Autodesk Inventor part; units mm, degrees
ref_plane "YZ Plane" through (0, 0, 0) normal (1, 0, 0) x (0, 1, 0)
ref_plane "XZ Plane" through (0, 0, 0) normal (0, 1, 0) x (-1, 0, 0)
ref_plane "XY Plane" through (0, 0, 0) normal (0, 0, 1) x (1, 0, 0)
sketch "スケッチ2" plane through (0, 0, 0) normal (0, 1, 0) x (-1, 0, 0)
  circle A0 centre (0, 0) radius 1.5
  circle A1 centre (0, 0) radius 2.25
  circle A2 centre (0, 0) radius 2.75
  line L0 (2.75, 2.75) -> (-2.75, -2.75) construction
  line L1 (1.0066, 4.2082) -> (1.0066, -4.7182) construction
  line L2 (3.3819, 0) -> (-4.1959, 0) construction
  line L3 (-2.75, -1.5877) -> (0, -3.1754)
  line L4 (-2.1903, -1.9109) -> (0.8771, -1.9109) construction
  line L5 (-2.75, 0) -> (-2.75, -1.5877)
  line L6 (0, 3.6036) -> (0, -4.7182) construction
  line L7 (-2.75, 1.5877) -> (0, 3.1754)
  line L8 (-2.75, 0) -> (-2.75, 1.5877)
  line L9 (2.75, -1.5877) -> (0, -3.1754)
  line L10 (2.75, 0) -> (2.75, -1.5877)
  line L11 (2.75, 1.5877) -> (0, 3.1754)
  line L12 (2.75, 0) -> (2.75, 1.5877)
  dimension "d8" = 5.5
  dimension "d6" = 3
  dimension "d7" = 4.5
  dimension "d12" = 30
extrude "押し出し1" add sketch "スケッチ2" against normal blind 0.7 contours A1
extrude "押し出し2" add sketch "スケッチ2" along normal blind 2.1 contours A1 | A2 | L10 L9 A2 | A2 L11 L12 | A2 L7 L11 | L9 L3 A2 | A2 L8 L7 | L3 L5 A2
chamfer "面取り1" distance 0.2 angle 45 6 edges at (2.75, 1.05, -1.5877) (0, 1.05, -3.1754) (-2.75, 1.05, -1.5877) (-2.75, 1.05, 1.5877) (0, 1.05, 3.1754) (2.75, 1.05, 1.5877)
chamfer "面取り2" distance 0.2 angle 45 6 edges at (2.6634, 2.1, -1.5377) (0, 2.1, -3.0754) (-2.6634, 2.1, -1.5377) (-2.6634, 2.1, 1.5377) (0, 2.1, 3.0754) (2.6634, 2.1, 1.5377)
thread "ねじ1"
properties part number "S3-07-3W" material "ステンレス鋼 AISI 304"
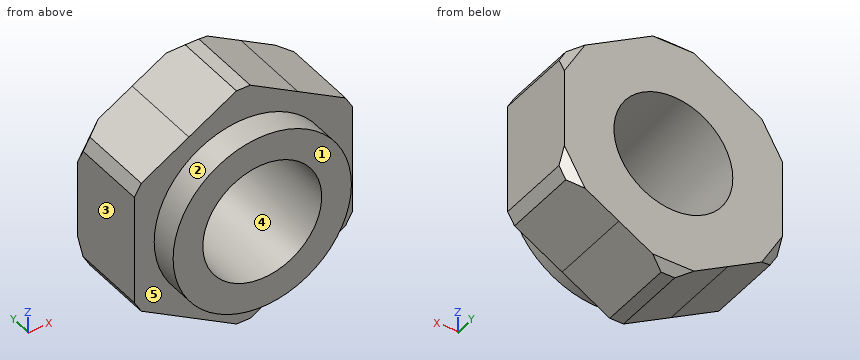
CAD build for the part. Positions are in the model's coordinates, mm. Face numbers are marked on the shaded views. A direction names the side the tool comes from. Coordinates: 2 decimals unless noted, no trailing zeros. Order: outer loops, then holes, each group sorted by start corner. A loop starts at its lowest first (then second) coordinate and runs counter-clockwise, first axis right, second up. Notation, with made-up numbers: (30.25, 31) - (76.25, 31) arc R19 cw to (76.25, 67) - close; hole circle Ø2 at (19, 43.25). An arc over 180 degrees is marked (long way). Use a Markdown table: item, result. Add a question column.
(1) Saw through at C-C (y = 0.7). Give the cut face in (x, z).
(2) Pull direction X, two halves, no side cores. Call the marked faces 3, 4 and 5: +X half, -X half, draft (parallel to the pull), parting line (faces both ways), or undercut.
(3) Drill centre lines: line 1 along Z through (x, y) = (0, 1.15); line 2 along Z through (x, y) = (0, -0.05); line 3 along X through (y, z) = (1.6, -0.25). Where is each one in solid material? Low to high. Write a range as [from, to].
(4) Saw through at A-A (x = 0). Give the cut face in (y, z).
(5) Which spindle directions (+Z, -Z, +X, -X, +Y, -Y) get a long thin tool onto all of the face, cutting with end or side? Do the marked faces 1 and 2. Say none if no direction does.
(6) Saw through at B-B (z = 0). Give the cut face in (x, y).
(7) Saw through at D-D (x = 0.65). Give the cut face in (y, z), then the cut area to 3 significant figures.
Solved:
| question | item | result |
|---|---|---|
| 1 | outline | (-2.75, -1.39) - (-2.58, -1.69) - (-0.17, -3.08) - (0.17, -3.08) - (2.58, -1.69) - (2.75, -1.39) - (2.75, 1.39) - (2.58, 1.69) - (0.17, 3.08) - (-0.17, 3.08) - (-2.58, 1.69) - (-2.75, 1.39) - close; hole circle Ø3 at (0, 0) |
| 2 | face 3 | -X half |
| 2 | face 4 | undercut |
| 2 | face 5 | draft |
| 3 | line 1 | z = [-3.08, -1.5], [1.5, 3.08] |
| 3 | line 2 | z = [-2.25, -1.5], [1.5, 2.25] |
| 3 | line 3 | x = [-2.75, -1.48], [1.48, 2.75] |
| 4 | outline | (-0.7, -2.25) - (0, -2.25) - (0, -3.08) - (1.9, -3.08) - (2.1, -2.88) - (2.1, -1.5) - (-0.7, -1.5) - close; (-0.7, 1.5) - (2.1, 1.5) - (2.1, 2.88) - (1.9, 3.08) - (0, 3.08) - (0, 2.25) - (-0.7, 2.25) - close |
| 5 | face 1 | +Z, -Z, +X, -X, -Y |
| 5 | face 2 | -Y |
| 6 | outline | (-2.75, 0) - (-2.25, 0) - (-2.25, -0.7) - (-1.5, -0.7) - (-1.5, 2.1) - (-2.75, 2.1) - close; (1.5, -0.7) - (2.25, -0.7) - (2.25, 0) - (2.75, 0) - (2.75, 2.1) - (1.5, 2.1) - close |
| 7 | outline | (-0.7, -2.15) - (0, -2.15) - (0, -2.8) - (2.1, -2.8) - (2.1, -1.35) - (-0.7, -1.35) - close; (-0.7, 1.35) - (2.1, 1.35) - (2.1, 2.8) - (0, 2.8) - (0, 2.15) - (-0.7, 2.15) - close |
| 7 | area | 7.21 mm² |
